For this review, take the finished solid that the model builds, in its own axes (mm). A direction names the side the tool comes from. Coordinates: 2 decimals unless noted, no trailing zeros. Order: outer loops, then holes, each group sorted by start corner. A loop starts at its lowest first (then second) coordinate and runs counter-clockwise, first axis right, second up.
from build123d import *

# Parameters (mm, degrees)
CROQUIS1_R              = 1
SALIENTE_EXTRUIR1_DEPTH = 15
SALIENTE_EXTRUIR2_START = -3
CROQUIS2_R              = 1
SALIENTE_EXTRUIR2_DEPTH = 3
CROQUIS3_R              = 1
SALIENTE_EXTRUIR3_DEPTH = 3


with BuildPart() as part:
    # Croquis1 → Saliente-Extruir1 (new body)
    with BuildSketch(Plane(origin=(0, 0, 0), x_dir=(1, 0, 0), z_dir=(0, 1, 0))):
        with BuildLine():
            Line((-2.5, -7.5), (-2.5, 7.5))
            ThreePointArc((-2.5, 7.5), (0, 10), (2.5, 7.5))
            Line((2.5, 7.5), (2.5, -7.5))
            ThreePointArc((2.5, -7.5), (0, -10), (-2.5, -7.5))
        make_face()
        with Locations(Location((0, 7.5, 0), (0, 0, 270))):
            Circle(CROQUIS1_R, mode=Mode.SUBTRACT)
        with Locations(Location((0, -7.5, 0), (0, 0, 270))):
            Circle(CROQUIS1_R, mode=Mode.SUBTRACT)
    extrude(amount=SALIENTE_EXTRUIR1_DEPTH)

    # Croquis2 → Saliente-Extruir2 (add)
    with BuildSketch(Plane(origin=(0, 6, 0), x_dir=(-1, 0, 0), z_dir=(0, 1, 0)).offset(SALIENTE_EXTRUIR2_START)):
        with BuildLine():
            Line((-2.5, -7.5), (-2.5, 0))
            Line((-2.5, 0), (-8.769008438, -4.577066004))
            ThreePointArc((-8.769008438, -4.577066004), (-9.852087129, -7.930375734), (-7, -10))
            Line((-7, -10), (0, -10))
            ThreePointArc((0, -10), (-1.767766953, -9.267766953), (-2.5, -7.5))
        make_face()
        with Locations(Location((-7, -7, 0), (0, 0, 90))):
            Circle(CROQUIS2_R, mode=Mode.SUBTRACT)
    extrude(amount=SALIENTE_EXTRUIR2_DEPTH)

    # Croquis3 → Saliente-Extruir3 (add)
    with BuildSketch(Plane(origin=(0, 9, 0), x_dir=(-1, 0, 0), z_dir=(0, 1, 0))):
        with BuildLine():
            Line((-7, -10), (0, -10))
            ThreePointArc((0, -10), (-1.767766953, -9.267766953), (-2.5, -7.5))
            Line((-2.5, -7.5), (-2.5, 0))
            Line((-2.5, 0), (-8.769008438, -4.577066004))
            ThreePointArc((-8.769008438, -4.577066004), (-9.852087129, -7.930375734), (-7, -10))
        make_face()
        with Locations(Location((-7, -7, 0), (0, 0, 90))):
            Circle(CROQUIS3_R, mode=Mode.SUBTRACT)
    extrude(amount=SALIENTE_EXTRUIR3_DEPTH)


solid = part.part
1. Take a section at A-A, the plane x = 5.5. Give the boundary of the cut face in (y, z).
Answer below:
outline: (3, -10) - (6, -10) - (6, -2.19) - (3, -2.19) - close; (9, -10) - (12, -10) - (12, -2.19) - (9, -2.19) - close
2. Machinability: for faces 1 (the face through (5.591, 10.479, -2.256)), 2 (the face through (2.5, 7, 2)), 3 (the face through (-0.91, 7.4, -9.83)), which of the approach directions +Z, -Z, +X, -X, +Y, -Y give a long, thin tool a straight path to every point of the face, cutting with its end or side? Answer none if there is none.
Answer below:
face 1: +Z, +X, +Y, -Y
face 2: +Z, +X
face 3: -Z
3. Take a section at B-B, the plane z = -8.25. Give the boundary of the cut face in (x, y).
Answer below:
outline: (-2.38, 0) - (-0.66, 0) - (-0.66, 15) - (-2.38, 15) - close; (0.66, 0) - (2.38, 0) - (2.38, 3) - (9.73, 3) - (9.73, 6) - (2.38, 6) - (2.38, 9) - (9.73, 9) - (9.73, 12) - (2.38, 12) - (2.38, 15) - (0.66, 15) - close
4. Take a section at C-C, the plane y = 9.75. Give the boundary of the cut face in (x, z), plus the area to 3 significant figures.
Answer below:
outline: (-2.5, -7.5) arc R2.5 ccw to (0, -10) - (7, -10) arc R3 ccw to (8.77, -4.58) - (2.5, 0) - (2.5, 7.5) arc R2.5 ccw to (-2.5, 7.5) - close; hole circle Ø2 at (0, -7.5); hole circle Ø2 at (0, 7.5); hole circle Ø2 at (7, -7)
area: 139 mm2
5. The part is to be moulded in two halves that separate along Z. For faces 4 (the face through (9.87, 4.48, -7.88)), 5 (the face through (0, 15, 0)), 6 (the face through (-0.6, 7.4, 6.7)), say which applies: +Z half, -Z half, draft (parallel to the pull), parting line (faces both ways), or undercut.
Answer below:
face 4: parting line
face 5: draft
face 6: undercut
6. Take a section at D-D, the plane x = 1.5. Give the boundary of the cut face in (y, z).
Answer below:
outline: (0, -9.5) - (3, -9.5) - (3, -10) - (6, -10) - (6, -9.5) - (9, -9.5) - (9, -10) - (12, -10) - (12, -9.5) - (15, -9.5) - (15, 9.5) - (0, 9.5) - close
7. To check wall thickness, follow L1, parallel to X at y = 9.5, z = 7.5; L2, parallel to Z at x = -0.5, y = 1.25; L3, parallel to Z at x = 0.5, y = 11.75. State the ranges of each line that lie inside material, in increasing order.
Answer below:
L1: x = -2.5 to -1, 1 to 2.5
L2: z = -9.95 to -8.37, -6.63 to 6.63, 8.37 to 9.95
L3: z = -10 to -8.37, -6.63 to 6.63, 8.37 to 9.95
8. Clearance check with flat-ended pins moving along their axes: pin 1 Ø3 at (x, z) = (4.5, -7) entering from -Y; pin 2 Ø8 at (y, z) = (5, 7.5) entering from +X; pin 3 Ø5 at (x, z) = (7.5, -5) entering from +Y; pin 4 Ø1.6 at (x, z) = (0, -7.5) entering from +Y. State where each tip first meets the part, or that it passes through.
Answer below:
pin 1: stops at y = 3
pin 2: stops at x = 2.5
pin 3: stops at y = 12
pin 4: passes through
